Can you work these out from the model? Positions are in its coordinate system, mm. A direction names the side the tool comes from. Coordinates: 2 decimals unless noted, no trailing zeros. Loops run counter-clockwise (first coordinate to the right, second up) from the corner with the lowest first, then second, coordinate; pieces in that order, holes last.
```python
from build123d import *

# Parameters (mm, degrees)
ESBO_O2_R                = 2.5
RESSALTO_EXTRUS_O1_DEPTH = 29
ESBO_O3_R                = 4
CORTE_EXTRUS_O1_DEPTH    = 43.026777178


with BuildPart() as part:
    # Esboço2 → Ressalto-extrusão1 (new body)
    with BuildSketch(Plane.XY):
        with BuildLine():
            Line((-27.5, -3.5), (-27.5, 3.5))
            ThreePointArc((-27.5, 3.5), (-26.621320344, 5.621320344), (-24.5, 6.5))
            Line((-24.5, 6.5), (24.5, 6.5))
            ThreePointArc((24.5, 6.5), (26.621320344, 5.621320344), (27.5, 3.5))
            Line((27.5, 3.5), (27.5, -3.5))
            ThreePointArc((27.5, -3.5), (26.621320344, -5.621320344), (24.5, -6.5))
            Line((24.5, -6.5), (-24.5, -6.5))
            ThreePointArc((-24.5, -6.5), (-26.621320344, -5.621320344), (-27.5, -3.5))
        make_face()
        with Locations(Location((-21, 0, 0), (0, 0, 180))):
            Circle(ESBO_O2_R, mode=Mode.SUBTRACT)
        with Locations(Location((21, 0, 0), (0, 0, 180))):
            Circle(ESBO_O2_R, mode=Mode.SUBTRACT)
    extrude(amount=RESSALTO_EXTRUS_O1_DEPTH)

    # Esboço3 → Corte-extrusão1 (cut, through all)
    with BuildSketch(Plane.XZ.offset(6.5)):
        with Locations((0, 16)):
            Circle(ESBO_O3_R)
        with BuildLine():
            Line((-27.5, 29), (-13.643156348, 29))
            Line((-13.643156348, 29), (-13.643156348, 9.087055385))
            ThreePointArc((-13.643156348, 9.087055385), (-14.521836004, 6.965735042), (-16.643156348, 6.087055385))
            Line((-16.643156348, 6.087055385), (-27.5, 6.087055385))
            Line((-27.5, 6.087055385), (-27.5, 29))
        make_face()
        with BuildLine():
            Line((27.5, 6.087055385), (16.643156348, 6.087055385))
            ThreePointArc((16.643156348, 6.087055385), (14.521836004, 6.965735042), (13.643156348, 9.087055385))
            Line((13.643156348, 9.087055385), (13.643156348, 29))
            Line((13.643156348, 29), (27.5, 29))
            Line((27.5, 29), (27.5, 6.087055385))
        make_face()
    extrude(amount=-CORTE_EXTRUS_O1_DEPTH, mode=Mode.SUBTRACT)


solid = part.part
```
Item 1: Suppose I cut it at D-D, the plane y = 5. Please give me the cut outline in (x, z), plus the area to 3 significant figures.
Results are:
outline: (-27.1, 0) - (27.1, 0) - (27.1, 6.09) - (16.64, 6.09) arc R3 cw to (13.64, 9.09) - (13.64, 29) - (-13.64, 29) - (-13.64, 9.09) arc R3 cw to (-16.64, 6.09) - (-27.1, 6.09) - close; hole circle Ø8 at (0, 16)
area: 909 mm2
Item 2: Suppose I cut it at A-A, the plane x = -21. Please give me the cut outline in (y, z), plus the area to 3 significant figures.
Results are:
outline: (-6.5, 0) - (-2.5, 0) - (-2.5, 6.09) - (-6.5, 6.09) - close; (2.5, 0) - (6.5, 0) - (6.5, 6.09) - (2.5, 6.09) - close
area: 48.7 mm2
Item 3: I need wall thicknesses on line 1 along Y through (x, z) = (-21, 4.5); line 2 along Z through (x, y) = (-22.5, 5.25); line 3 along X through (y, z) = (-3.5, 11.75). Which ranges of each line are inside material? Lowest first, please.
Results are:
line 1: y = -6.5 to -2.5, 2.5 to 6.5
line 2: z = 0 to 6.09
line 3: x = -13.64 to 13.64
Item 4: On a 3-axis mill with a long thin cutter (end or side, diameter ignored), from which of +Z, -Z, +X, -X, +Y, -Y can I reach the whole of each face in a straight line? I mean faces 1 (the face through (-0.521, -0.091, 19.966)), 2 (the face through (13.643, 0, 19)), 3 (the face through (-23, -2, 6.087)). Say none if no direction works.
Results are:
face 1: +Y, -Y
face 2: +Z, +X, +Y, -Y
face 3: +Z, -X, +Y, -Y
Item 5: I'm going to push flat-ended pins straight in: P1, Ø3, axis at x = -16, z = 12.5, coming from the -Y side; P2, Ø1, axis at y = 2.5, z = 8.5, coming from the +X side; P3, Ø12, axis at x = 18, z = 18.5, coming from the +Y side; P4, Ø1, axis at y = 4.5, z = 3.5, coming from the -X side. Where does each tip first touch, or does it pass through?
Results are:
P1: passes through
P2: stops at x = 13.85
P3: stops at y = 6.5
P4: stops at x = -27.46
Item 6: Suppose I cut it at C-C, the plane z = 16. Please give me the cut outline in (x, y), plus the area to 3 significant figures.
Results are:
outline: (-13.64, -6.5) - (-4, -6.5) - (-4, 6.5) - (-13.64, 6.5) - close; (4, -6.5) - (13.64, -6.5) - (13.64, 6.5) - (4, 6.5) - close
area: 251 mm2
Item 7: We'd pull the mould along X, two halves only. Please class faces 4 (the face through (-18.5, -0.1, 3)), 5 (the face through (-13.643, 0, 19)), 6 (the face through (26.6, 5.64, 3)), 7 (the face through (23, -2, 6.087)): +X half, -X half, draft (parallel to the pull), parting line (faces both ways), or undercut.
Results are:
face 4: undercut
face 5: -X half
face 6: +X half
face 7: draft
Item 8: Suppose I cut it at B-B, the plane y = 0.75. Please give me the cut outline in (x, z).
Results are:
outline: (-27.5, 0) - (-23.38, 0) - (-23.38, 6.09) - (-27.5, 6.09) - close; (-18.62, 0) - (18.62, 0) - (18.62, 6.09) - (16.64, 6.09) arc R3 cw to (13.64, 9.09) - (13.64, 29) - (-13.64, 29) - (-13.64, 9.09) arc R3 cw to (-16.64, 6.09) - (-18.62, 6.09) - close; (23.38, 0) - (27.5, 0) - (27.5, 6.09) - (23.38, 6.09) - close; hole circle Ø8 at (0, 16)
